```python
from build123d import *

# Parameters (mm, degrees)
SKETCH1_R           = 2.032
SKETCH1_R_2         = 2.54
BOSS_EXTRUDE1_DEPTH = 4.064


with BuildPart() as part:
    # Sketch1 → Boss-Extrude1 (new body)
    with BuildSketch(Plane.XY):
        with BuildLine():
            Line((0, 0), (0, 10.667831766))
            ThreePointArc((0, 10.667831766), (1.08596755, 14.588395494), (4.034335943, 17.391477598))
            Line((4.034335943, 17.391477598), (39.755950307, 36.44151561))
            ThreePointArc((39.755950307, 36.44151561), (41.504009214, 37.112976763), (43.363043022, 37.337839648))
            Line((43.363043022, 37.337839648), (79.046414123, 37.237491906))
            Line((79.046414123, 37.237491906), (86.410224142, 29.873681887))
            Line((86.410224142, 29.873681887), (86.410224142, 24.325303591))
            Line((86.410224142, 24.325303591), (30.226, 0))
            Line((30.226, 0), (0, 0))
        make_face()
        with Locations((6.35, 6.35)):
            Circle(SKETCH1_R, mode=Mode.SUBTRACT)
        with Locations((23.876, 6.35)):
            Circle(SKETCH1_R, mode=Mode.SUBTRACT)
        with Locations((55.230707363, 25.085785264)):
            Circle(SKETCH1_R_2, mode=Mode.SUBTRACT)
    extrude(amount=-BOSS_EXTRUDE1_DEPTH)


solid = part.part
```
Here's how the part is built. I have some questions about the finished solid (model axes, mm). Round coordinates to 2 decimals unless told otherwise and drop trailing zeros. Write each loop counter-clockwise with the first axis right and the second up, starting at its lowest first coordinate (ties: lowest second). Pieces come first, ordered by that corner, then holes.
Q1. Will this pin go through, and if not, where does the flat tip stop? P1, Ø2, axis at y = 31.5, z = -3, coming from the -X side.
Q2. If we section it at C-C on z = -1: Write out the boundary of the cut face in (x, y), plus the area to 3 significant figures.
Q3. If we section it at A-A on x = 6.35: Write out the boundary of the cut face in (y, z).
Q4. If we section it at D-D on x = 39: Write out the boundary of the cut face in (y, z).
Q5. If we mould it in two halves opening along X, with no side actions, what happens to faces 1 (the flat face through (58.711, 12.333, -2.004)), 2 (the cylindrical face through (52.693, 25.197, -2.004)), 3 (the flat face through (44, 19, -4.064)), 4 (the cylindrical face through (4.32, 6.44, -2))? For each: +X half, -X half, draft (parallel to the pull), parting line (faces both ways), or undercut.
Q6. Please list where these lines run through material, in increasing order: probe 1 along X at (y, z) = (7, -2.1); probe 2 along Y at (x, z) = (6.35, -2.8); probe 3 along Y at (x, z) = (67, -3.85).
Q7. If we section it at B-B on y = 6.35: Write out the boundary of the cut face in (x, z), plus the area to 3 significant figures.
Answer below:
1. P1: stops at x = 28.61
2. outline: (0, 0) - (30.23, 0) - (86.41, 24.33) - (86.41, 29.87) - (79.05, 37.24) - (43.36, 37.34) arc R7.62 ccw to (39.76, 36.44) - (4.03, 17.39) arc R7.62 ccw to (0, 10.67) - close; hole circle Ø4.06 at (6.35, 6.35); hole circle Ø4.06 at (23.88, 6.35); hole circle Ø5.08 at (55.23, 25.09)
2. area: 2,010 mm2
3. outline: (0, -4.06) - (4.32, -4.06) - (4.32, 0) - (0, 0) - close; (8.38, -4.06) - (18.63, -4.06) - (18.63, 0) - (8.38, 0) - close
4. outline: (3.8, -4.06) - (36.04, -4.06) - (36.04, 0) - (3.8, 0) - close
5. face 1: +X half
5. face 2: undercut
5. face 3: draft
5. face 4: undercut
6. probe 1: x = 0 to 4.42, 8.28 to 21.95, 25.8 to 46.39
6. probe 2: y = 0 to 4.32, 8.38 to 18.63
6. probe 3: y = 15.92 to 37.27
7. outline: (0, -4.06) - (4.32, -4.06) - (4.32, 0) - (0, 0) - close; (8.38, -4.06) - (21.84, -4.06) - (21.84, 0) - (8.38, 0) - close; (25.91, -4.06) - (44.89, -4.06) - (44.89, 0) - (25.91, 0) - close
7. area: 149 mm2
